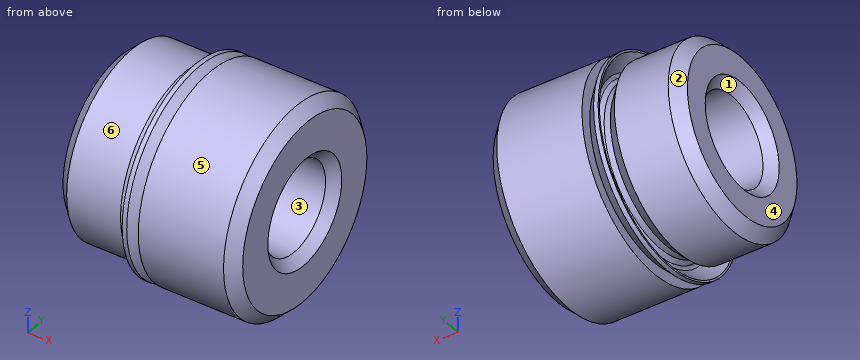
Autodesk Inventor part; units mm, degrees
ref_plane "lovra_XY" through (8.3312, 0, 0) normal (1, 0, 0) x (0, 1, 0)
ref_plane "lovra_YZ" through (8.3312, 0, 0) normal (0, 1, 0) x (0, 0, 1)
ref_plane "lovra_ZX" through (8.3312, 0, 0) normal (0, 0, 1) x (1, 0, 0)
sketch "Sketch_1" plane through (0, 0, 0) normal (0, 0, 1) x (1, 0, 0)
  line L0 (8.3312, 0) -> (0, 0)
  line L1 (0, 0) -> (0, 3.5751)
  line L2 (0, 3.5751) -> (0.508, 4.0831)
  line L3 (0.508, 4.0831) -> (2.9083, 4.0831)
  line L4 (2.9083, 4.0831) -> (3.4671, 3.5242)
  line L5 (3.4671, 3.5242) -> (4.0259, 3.5242)
  line L6 (4.0259, 3.5242) -> (4.0259, 4.5593)
  line L7 (4.0259, 4.5593) -> (7.8232, 4.5593)
  line L8 (7.8232, 4.5593) -> (8.3312, 4.0513)
  line L9 (8.3312, 4.0513) -> (8.3312, 0)
  line L10 (8.3312, 0) -> (0, 0)
revolve "Revolution1" add sketch "Sketch_1" angle 360 about axis through (8.3312, 0, 0) along (1, 0, 0)
sketch "Sketch_2" plane through (0, 0, 0) normal (0, 0, 1) x (1, 0, 0)
  line L0 (8.3312, 0) -> (0, 0)
  line L1 (0, 0) -> (0, 2.413)
  line L2 (0, 2.413) -> (0.4293, 1.9837)
  line L3 (0.4293, 1.9837) -> (7.9019, 1.9837)
  line L4 (7.9019, 1.9837) -> (8.3312, 2.413)
  line L5 (8.3312, 2.413) -> (8.3312, 0)
  line L6 (8.3312, 0) -> (0, 0)
revolve "Revolution2" cut sketch "Sketch_2" angle 360 about axis through (8.3312, 0, 0) along (1, 0, 0)
thread "Thread1"
sketch "Sketch_24" plane through (0, 0, 0) normal (0, 0, 1) x (1, 0, 0)
  line L0 (4.0259, 0) -> (3.4671, 0)
  line L1 (3.3065, 4.5593) -> (3.3065, 4.4751)
  line L2 (3.3065, 4.4751) -> (3.9121, 3.8695)
  arc A0 (3.9121, 3.6899) -> (3.9121, 3.8695) centre (3.8223, 3.7797) ccw
  line L3 (3.9121, 3.6899) -> (3.7465, 3.5242)
  line L4 (3.7465, 3.5242) -> (3.4671, 3.5242)
  line L5 (3.4671, 3.5242) -> (3.4671, 3.2702)
  line L6 (3.4671, 3.2702) -> (4.0259, 3.2702)
  line L7 (4.0259, 3.2702) -> (4.0259, 4.0431)
  line L8 (4.0259, 4.0431) -> (3.5097, 4.5593)
  line L9 (3.5097, 4.5593) -> (3.3065, 4.5593)
revolve "Revolution3" add sketch "Sketch_24" angle 360 about axis through (4.0259, 0, 0) along (1, 0, 0)
ref_plane "lovra_XY" through (8.3312, 0, 0) normal (1, 0, 0) x (0, 1, 0)
ref_plane "lovra_YZ" through (8.3312, 0, 0) normal (0, 1, 0) x (0, 0, 1)
ref_plane "lovra_ZX" through (8.3312, 0, 0) normal (0, 0, 1) x (1, 0, 0)
ref_plane "lovra1_XY" through (8.3312, 0, 0) normal (1, 0, 0) x (0, 0, -1)
ref_plane "lovra1_YZ" through (8.3312, 0, 0) normal (0, 0, -1) x (0, 1, 0)
ref_plane "lovra1_ZX" through (8.3312, 0, 0) normal (0, 1, 0) x (1, 0, 0)
ref_plane "lovra2_XY" through (8.3312, 0, 0) normal (1, 0, 0) x (0, 0, -1)
ref_plane "lovra2_YZ" through (8.3312, 0, 0) normal (0, 0, -1) x (0, 1, 0)
ref_plane "lovra2_ZX" through (8.3312, 0, 0) normal (0, 1, 0) x (1, 0, 0)
ref_plane "lovra21_XY" through (0, 0, 5.2705) normal (1, 0, 0) x (0, 0, -1)
ref_plane "lovra21_YZ" through (0, 0, 5.2705) normal (0, 0, -1) x (0, 1, 0)
ref_plane "lovra21_ZX" through (0, 0, 5.2705) normal (0, 1, 0) x (1, 0, 0)
ref_plane "lovra22_XY" through (0, 0, -5.2705) normal (1, 0, 0) x (0, 0, -1)
ref_plane "lovra22_YZ" through (0, 0, -5.2705) normal (0, 0, -1) x (0, 1, 0)
ref_plane "lovra22_ZX" through (0, 0, -5.2705) normal (0, 1, 0) x (1, 0, 0)
ref_plane "lovra3_XY" through (8.3312, 0, 0) normal (1, 0, 0) x (0, 0, -1)
ref_plane "lovra3_YZ" through (8.3312, 0, 0) normal (0, 0, -1) x (0, 1, 0)
ref_plane "lovra3_ZX" through (8.3312, 0, 0) normal (0, 1, 0) x (1, 0, 0)
ref_plane "olen_XY" through (8.3312, 0, 0) normal (1, 0, 0) x (0, 0, -1)
ref_plane "olen_YZ" through (8.3312, 0, 0) normal (0, 0, -1) x (0, 1, 0)
ref_plane "olen_ZX" through (8.3312, 0, 0) normal (0, 1, 0) x (1, 0, 0)
ref_plane "to_mounting_bracket_XY" through (13.5509, 0, 0) normal (1, 0, 0) x (0, 0, -1)
ref_plane "to_mounting_bracket_YZ" through (13.5509, 0, 0) normal (0, 0, -1) x (0, 1, 0)
ref_plane "to_mounting_bracket_ZX" through (13.5509, 0, 0) normal (0, 1, 0) x (1, 0, 0)
ref_plane "to_nut_XY" through (0, 0, 0) normal (1, 0, 0) x (0, 0, -1)
ref_plane "to_nut_YZ" through (0, 0, 0) normal (0, 0, -1) x (0, 1, 0)
ref_plane "to_nut_ZX" through (0, 0, 0) normal (0, 1, 0) x (1, 0, 0)
ref_plane "to_pin_XY" through (18.2626, 0, 0) normal (0, 0, 1) x (1, 0, 0)
ref_plane "to_pin_YZ" through (18.2626, 0, 0) normal (1, 0, 0) x (0, 1, 0)
ref_plane "to_pin_ZX" through (18.2626, 0, 0) normal (0, 1, 0) x (0, 0, 1)
ref_plane "to_screw_XY" through (9.525, 0, 0) normal (0, 1, 0) x (1, 0, 0)
ref_plane "to_screw_YZ" through (9.525, 0, 0) normal (1, 0, 0) x (0, 0, -1)
ref_plane "to_screw_ZX" through (9.525, 0, 0) normal (0, 0, -1) x (0, 1, 0)
ref_plane "to_tube_XY" through (3.4671, 0, 0) normal (1, 0, 0) x (0, 0, -1)
ref_plane "to_tube_YZ" through (3.4671, 0, 0) normal (0, 0, -1) x (0, 1, 0)
ref_plane "to_tube_ZX" through (3.4671, 0, 0) normal (0, 1, 0) x (1, 0, 0)
properties part number "0070000_rear_head"
Can you work these out from the model? Positions are in its coordinate system, mm. Face numbers are marked on the shaded views. A direction names the side the tool comes from. Round coordinates to 2 decimals unless told otherwise and drop trailing zeros. Loops run counter-clockwise (first coordinate to the right, second up) from the corner with the lowest first, then second, coordinate; pieces in that order, holes last.
Item 1: If we mould it in two halves opening along Y, with no side actions, what happens to the marked faces 1, 2, 3 and 4? For each: +Y half, -Y half, draft (parallel to the pull), parting line (faces both ways), or undercut.
Item 2: Which directions (+Z, -Z, +X, -X, +Y, -Y) give clear straight access to the entire face, cutting with the end or side of a thin tool? Please do the marked faces 5 and 6.
Item 3: Suppose I cut it at B-B, the plane x = 2.25. Write out the boundary of the cut face in (y, z).
Item 4: Will these pins go through, and if not, where does the flat tip stop? pin 1 Ø3 at (x, z) = (3, -2.5) entering from +Y; pin 2 Ø2.5 at (y, z) = (0, 0) entering from +X; pin 3 Ø3 at (x, y) = (2.5, 2.5) entering from -Z.
Item 5: Suppose I cut it at A-A, the plane x = 5.5. Write out the boundary of the cut face in (y, z), then the cut area to 3 significant figures.
Item 6: Please list where these lines run through material, in increasing order: L1, parallel to Z at x = 5.5, y = 0; L2, parallel to Z at x = 2, y = -1.25; L3, parallel to Y at x = 1, z = -1.
Reported:
1. face 1: undercut
1. face 2: parting line
1. face 3: undercut
1. face 4: draft
2. face 5: +X, -X
2. face 6: -X
3. outline: circle Ø8.17 at (0, 0); hole circle Ø3.97 at (0, 0)
4. pin 1: stops at y = 4.44
4. pin 2: passes through
4. pin 3: stops at z = -4.39
5. outline: circle Ø9.12 at (0, 0); hole circle Ø3.97 at (0, 0)
5. area: 52.9 mm2
6. L1: z = -4.56 to -1.98, 1.98 to 4.56
6. L2: z = -3.89 to -1.54, 1.54 to 3.89
6. L3: y = -3.96 to -1.71, 1.71 to 3.96
